Geometry check sheet. Reference: the model listing, model coordinates, mm. A direction names the side the tool comes from. Give positions to 0.01 mm unless a question says otherwise; leave off trailing zeros. Write each loop counter-clockwise with the first axis right and the second up, starting at its lowest first coordinate (ties: lowest second). Pieces come first, ordered by that corner, then holes. Notation, with made-up numbers: (86.5, -19) -> (102.5, -19) arc R25 cw to (102.5, 4) -> close; hole circle Ø10 at (82.5, 32). An arc over 180 degrees is marked (long way). One line per item, written item: value.
from build123d import *

# Parameters (mm, degrees)
BOSS_EXTRUDE1_DEPTH                   = 76.2
TAP_DRILL_FOR_M3X0_5_TAP1_D           = 2.5
TAP_DRILL_FOR_M3X0_5_TAP1_CSINK_D     = 2.55
TAP_DRILL_FOR_M3X0_5_TAP1_CSINK_ANGLE = 90


with BuildPart() as part:
    # Sketch1 → Boss-Extrude1 (new body)
    with BuildSketch(Plane(origin=(0, 0, 0), x_dir=(1, 0, 0), z_dir=(0, 1, 0))):
        with BuildLine():
            Line((-44.247201079, 4.24119048), (-54.936217795, 4.24119048))
            Line((-54.936217795, 4.24119048), (-54.936217795, 0))
            Line((-54.936217795, 0), (-40.716846583, 0))
            ThreePointArc((-40.716846583, 0), (0, 40.716846583), (40.716846583, 0))
            Line((40.716846583, 0), (55.359579402, 0))
            Line((55.359579402, 0), (55.359579402, 4.24119048))
            Line((55.359579402, 4.24119048), (44.247201079, 4.24119048))
            ThreePointArc((44.247201079, 4.24119048), (0, 44.45), (-44.247201079, 4.24119048))
        make_face()
    extrude(amount=BOSS_EXTRUDE1_DEPTH)

    # Tap Drill for M3x0.5 Tap1 (through all)
    with Locations(Plane(origin=(50.171881224, 66.945390665, -4.24119048), x_dir=(-1, 0, 0), z_dir=(0, 0, -1))):
        with Locations((0, 0), (0.880500078, -59.713914359), (99.976781548, -59.713914359), (99.976781548, 0)):
            CounterSinkHole(TAP_DRILL_FOR_M3X0_5_TAP1_D / 2, TAP_DRILL_FOR_M3X0_5_TAP1_CSINK_D / 2, counter_sink_angle=TAP_DRILL_FOR_M3X0_5_TAP1_CSINK_ANGLE)


solid = part.part
1) Sectioned sample at D-D on x = -36. Record the cut outline in (y, z), plus the area to 3 significant figures.
Verdict:
outline: (0, -26.07) -> (76.2, -26.07) -> (76.2, -19.02) -> (0, -19.02) -> close
area: 537 mm^2
2) Tool access check on faces 1 (the cylindrical face through (-49.228, 65.836, -2.079)), 2 (the flat face through (-50, 38, -4.241)), 3 (the flat face through (50, 38, -4.241)). Record the directions out of +Z, -Z, +X, -X, +Y, -Y that give a thin tool (end or side, any length) a straight path to the whole face; none if there is none.
Verdict:
face 1: +Z, -Z
face 2: -Z, -X, +Y, -Y
face 3: -Z, +X, +Y, -Y
3) Sectioned sample at C-C on x = 0. Record the cut outline in (y, z), plus the area to 3 significant figures.
Verdict:
outline: (0, -44.45) -> (76.2, -44.45) -> (76.2, -40.72) -> (0, -40.72) -> close
area: 284 mm^2
4) Sectioned sample at A-A on y = 24.5. Record the cut outline in (x, z), plus the area to 3 significant figures.
Verdict:
outline: (-54.94, -4.24) -> (-44.25, -4.24) arc R44.45 ccw to (44.25, -4.24) -> (55.36, -4.24) -> (55.36, 0) -> (40.72, 0) arc R40.72 cw to (-40.72, 0) -> (-54.94, 0) -> close
area: 591 mm^2
5) Depth check by flat-ended pin: pin 1 Ø4 at (y, z) = (21.5, -17) entering from -X; pin 2 Ø12 at (x, y) = (-23.5, 66) entering from -Z; pin 3 Ø12 at (y, z) = (35, -15) entering from -X; pin 4 Ø1.5 at (x, y) = (50.17, 66.95) entering from -Z. Enter the tip coordinate at first touch or a pass-through.
Verdict:
pin 1: x = -41.84
pin 2: z = -40.86
pin 3: x = -43.53
pin 4: through
6) Sectioned sample at B-B on z = -20.5. Record the cut outline in (x, y).
Verdict:
outline: (-39.44, 0) -> (-35.18, 0) -> (-35.18, 76.2) -> (-39.44, 76.2) -> close; (35.18, 0) -> (39.44, 0) -> (39.44, 76.2) -> (35.18, 76.2) -> close
7) Mould release check, pull along X, two halves, no side actions. Record for faces 4 (the cylindrical face through (48.043, 7.286, -2.079)), 5 (the cylindrical face through (0.92, 37.57, -44.44)), 6 (the flat face through (0, 0, -42)): released by +X, released by -X, zero draft, split by the parting line, or undercut.
Verdict:
face 4: undercut
face 5: split by the parting line
face 6: zero draft
8) Scan lines: probe 1 along X at (y, z) = (66, -12); probe 2 along X at (y, z) = (58.5, -14); probe 3 along Z at (x, y) = (48.5, 51). Record each from-to range of solid material in increasing order.
Verdict:
probe 1: -42.8 to -38.91, 38.91 to 42.8
probe 2: -42.19 to -38.23, 38.23 to 42.19
probe 3: -4.24 to 0
